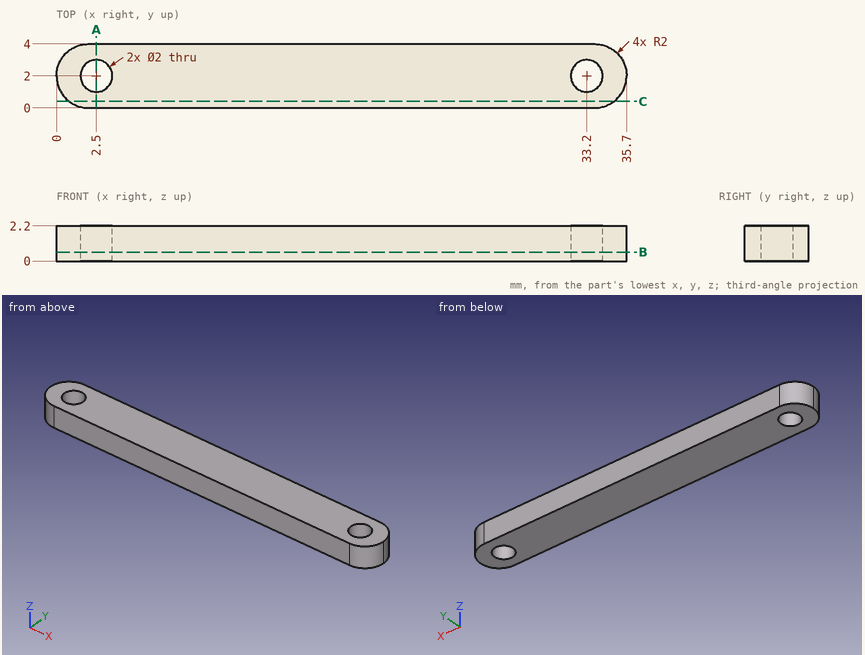
Input: dimensioned drawing with shaded views. Units: mm. Origin: part minimum x, y, z. Coordinates: 2 decimals unless noted, no trailing zeros. Order: outer loops, then holes, each group sorted by start corner. A loop starts at its lowest first (then second) coordinate and runs counter-clockwise, first axis right, second up. Notation, with made-up numbers: (10, 64.25) - (58, 64.25) arc R23 ccw to (58, 82.25) - close; hole circle Ø7 at (81.25, 9.5). An arc over 180 degrees is marked (long way). One line per item, written item: value.
1) Contact query for a flat-ended pin moving along its axis: pin 1 (1 mm diameter, centred on y = 0.5, z = 1, fed in from +X). Output: stop coordinate, or through.
Computed values:
pin 1: stops at x = 35.43
2) Ray query, line 1 (Y direction, x = 2.5, z = 0.85); line 2 (X direction, y = 1.45, z = 0.9) (1 decimal); line 3 (X direction, y = 2.5, z = 1.3). Return the intervals inside material, ascending. Write a range as [from, to].
Computed values:
line 1: y = [0, 1], [3, 4]
line 2: x = [0.1, 1.7], [3.3, 32.4], [34, 35.6]
line 3: x = [0.06, 1.63], [3.37, 32.33], [34.07, 35.64]
3) Cut plane B-B on z = 0.55. State how many separate pieces and enclosed holes the cut face has, plus the area to 3 significant figures.
Computed values:
separate pieces: 1
enclosed holes: 2
area: 133 mm^2
4) Cut plane A-A on x = 2.5. Output: boundary loops of the cut face in (y, z), plus the area to 3 significant figures.
Computed values:
outline: (0, 0) - (1, 0) - (1, 2.2) - (0, 2.2) - close; (3, 0) - (4, 0) - (4, 2.2) - (3, 2.2) - close
area: 4.40 mm^2
5) Cut plane C-C on y = 0.4. Output: boundary loops of the cut face in (x, z), plus the area to 3 significant figures.
Computed values:
outline: (0.8, 0) - (34.9, 0) - (34.9, 2.2) - (0.8, 2.2) - close
area: 75.0 mm^2
